Work out the finished part from the listing and answer in its coordinate system (mm). A direction names the side the tool comes from. Give positions to 0.01 mm unless a question says otherwise; leave off trailing zeros. Write each loop counter-clockwise with the first axis right and the second up, starting at its lowest first coordinate (ties: lowest second). Pieces come first, ordered by that corner, then holes. Notation, with made-up numbers: (0, 49.25) - (59, 49.25) arc R29 ccw to (59, 87.25) - close; hole circle Ø9 at (76, -34.5). An arc over 180 degrees is marked (long way). Write item = value, one per line.
from build123d import *

# Parameters (mm, degrees)
SKETCH1_R           = 10.5
BOSS_EXTRUDE1_DEPTH = 10
FILLET1_R           = 13
SKETCH8_R           = 1.6
SKETCH8_R_2         = 5
CUT_EXTRUDE5_DEPTH  = 122.553128346
SKETCH4_R           = 1.6
CUT_EXTRUDE6_DEPTH  = 10
FILLET2_R           = 1


with BuildPart() as part:
    # Sketch1 → Boss-Extrude1 (new body)
    with BuildSketch(Plane(origin=(0, 0, 0), x_dir=(1, 0, 0), z_dir=(0, 1, 0))):
        Polygon((108.646998451, -20), (108.646998451, 25.840472806), (-118.353001549, 25.840472806), (-118.353001549, -20), (-62.353001549, -20), (-62.353001549, 7.840472806), (52.646998451, 7.840472806), (52.646998451, -20), align=None)
        with Locations(Location((92.646998451, 0, 0), (0, 0, 270))):
            Circle(SKETCH1_R, mode=Mode.SUBTRACT)
        with Locations(Location((-102.353001549, 0, 0), (0, 0, 270))):
            Circle(SKETCH1_R, mode=Mode.SUBTRACT)
    extrude(amount=BOSS_EXTRUDE1_DEPTH)

    # Fillet1
    fillet1_edges = [part.edges().sort_by_distance(p)[0] for p in [
        (108.646998451, 5, -25.840472806),
        (108.646998451, 5, 20),
        (52.646998451, 5, 20),
        (52.646998451, 5, -7.840472806),
        (-62.353001549, 5, -7.840472806),
        (-62.353001549, 5, 20),
        (-118.353001549, 5, 20),
        (-118.353001549, 5, -25.840472806),
    ]]
    fillet(fillet1_edges, radius=FILLET1_R)

    # Sketch8 → Cut-Extrude5 (cut, through all)
    with BuildSketch(Plane(origin=(0, 10, 0), x_dir=(1, 0, 0), z_dir=(0, 1, 0))):
        with Locations(Location((-86.353001549, 0, 0), (0, 0, 90))):
            Circle(SKETCH8_R)
        with Locations(Location((-78.353001549, 0, 0), (0, 0, 90))):
            Circle(SKETCH8_R_2)
        with Locations(Location((-78.353001549, -8, 0), (0, 0, 90))):
            Circle(SKETCH8_R)
        with Locations(Location((-70.353001549, 0, 0), (0, 0, 90))):
            Circle(SKETCH8_R)
        with Locations(Location((-78.353001549, 8, 0), (0, 0, 90))):
            Circle(SKETCH8_R)
        with BuildLine():
            Line((-31.353001549, 23.590472806), (-26.353001549, 23.590472806))
            ThreePointArc((-26.353001549, 23.590472806), (-24.603001549, 21.840472806), (-26.353001549, 20.090472806))
            Line((-26.353001549, 20.090472806), (-31.353001549, 20.090472806))
            ThreePointArc((-31.353001549, 20.090472806), (-33.103001549, 21.840472806), (-31.353001549, 23.590472806))
        make_face()
        with BuildLine():
            Line((-31.353001549, 13.590472806), (-26.353001549, 13.590472806))
            ThreePointArc((-26.353001549, 13.590472806), (-24.603001549, 11.840472806), (-26.353001549, 10.090472806))
            Line((-26.353001549, 10.090472806), (-31.353001549, 10.090472806))
            ThreePointArc((-31.353001549, 10.090472806), (-33.103001549, 11.840472806), (-31.353001549, 13.590472806))
        make_face()
        with BuildLine():
            Line((21.646998451, 13.590472806), (16.646998451, 13.590472806))
            ThreePointArc((16.646998451, 13.590472806), (14.896998451, 11.840472806), (16.646998451, 10.090472806))
            Line((16.646998451, 10.090472806), (21.646998451, 10.090472806))
            ThreePointArc((21.646998451, 10.090472806), (23.396998451, 11.840472806), (21.646998451, 13.590472806))
        make_face()
        with BuildLine():
            Line((21.646998451, 23.590472806), (16.646998451, 23.590472806))
            ThreePointArc((16.646998451, 23.590472806), (14.896998451, 21.840472806), (16.646998451, 20.090472806))
            Line((16.646998451, 20.090472806), (21.646998451, 20.090472806))
            ThreePointArc((21.646998451, 20.090472806), (23.396998451, 21.840472806), (21.646998451, 23.590472806))
        make_face()
    extrude(amount=-CUT_EXTRUDE5_DEPTH, mode=Mode.SUBTRACT)

    # Sketch4 → Cut-Extrude6 (cut)
    with BuildSketch(Plane(origin=(0, 10, 0), x_dir=(1, 0, 0), z_dir=(0, 1, 0))):
        with Locations(Location((-4.853001549, 16.840472806, 0), (0, 0, 270))):
            Circle(SKETCH4_R)
    extrude(amount=-CUT_EXTRUDE6_DEPTH, mode=Mode.SUBTRACT)

    # Fillet2
    fillet2_edges = [part.edges().sort_by_distance(p)[0] for p in [
        (92.646998451, 10, -10.5),
        (-102.353001549, 10, -10.5),
    ]]
    fillet(fillet2_edges, radius=FILLET2_R)


solid = part.part
1. Find section A-A, the plane x = -35.5. Give the vertices of the cut face in (y, z), then the cut area to 3 significant figures.
Solution:
outline = (0, -25.84) - (10, -25.84) - (10, -7.84) - (0, -7.84) - close
area = 180 mm^2
2. For a pull along X with two mould halves and no side action, classify faces 4 (the flat face through (-3, 5, -25.84)), 5 (the flat face through (108.647, 5, -3)), 6 (the cylindrical face through (23.397, 5.07, -21.802)) as pulls with the +X half, pulls with the -X half, needs draft (parallel to the pull), parting line crosses it, or undercut.
Solution:
face_4 = needs draft
face_5 = pulls with the +X half
face_6 = undercut
3. A tool of negligible diameter and unlimited length cuts with its end or side. For faces 1 (the cylindrical face through (-58.444, 5.07, -4.133)), 2 (the flat face through (-29, 5, -10.09)), 3 (the cylindrical face through (-114.444, 5.07, -22.133)), from which of +Z, -Z, +X, -X, +Y, -Y can it reach the whole face along a straight path? Write none if from no direction.
Solution:
face_1 = +Z, +Y, -Y
face_2 = +Y, -Y
face_3 = -Z, -X, +Y, -Y
4. Find section B-B, the plane y = 2.5. Give the number of separate pieces and of enclosed holes in the cut face, then the cut area to 3 significant figures.
Solution:
separate_pieces = 1
enclosed_holes = 12
area = 6,140 mm^2
5. Given pin 1 (5.5 mm diameter, centred on x = 18.5, y = 5, fed in from +Z), flat-ended and moving along its own axis, determine where the tip first touches the part or whether it passes through.
Solution:
pin_1 = -7.84
6. Straight lines are drawn through the part: line 1 (X direction, y = 7, z = -12); line 2 (X direction, y = 5.5, z = 8); line 3 (X direction, y = 4.75, z = -21.5). For each, find the intervals that lie inside material, in ascending order.
Solution:
line_1 = -118.35 to -33.1, -24.61 to 14.9, 23.39 to 108.65
line_2 = -118.31 to -109.15, -95.55 to -79.95, -76.75 to -62.39, 52.69 to 85.85, 99.45 to 108.61
line_3 = -115.05 to -33.07, -24.64 to 14.93, 23.36 to 105.34
